Part model, mm, in its own coordinate system. Round coordinates to 2 decimals unless told otherwise and drop trailing zeros. Loops run counter-clockwise (first coordinate to the right, second up) from the corner with the lowest first, then second, coordinate; pieces in that order, holes last.
1) Probe line 1 (X direction, y = 1.2, z = 0); line 2 (Z direction, x = 2, y = 2.75); line 3 (X direction, y = 1.25, z = 5). List the from-to ranges inside material, lowest first.
2) Band-saw the part on C-C, the plane y = 2.5. State how many separate pieces and enclosed holes the cut face has, then the cut area to 3 significant figures.
3) Band-saw the part on A-A, the plane z = 0. Write the cut outline in (x, y).
4) Band-saw the part on D-D, the plane x = 30. Write the cut outline in (y, z).
5) Drop flat-ended pins along their axis: P1, Ø1, axis at y = 1, z = 8, coming from the -X side; P2, Ø0.9, axis at x = 87, y = 1.5, coming from the +Z side; P3, Ø0.9, axis at x = -1, y = 1, coming from the -Z side. Give the stop position or say it passes through.
6) Band-saw the part on B-B, the plane x = 0. Write the cut outline in (y, z), then the cut area to 3 significant figures.
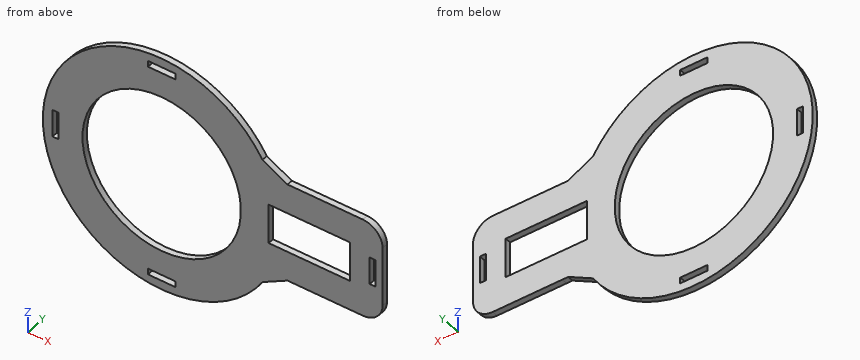
from build123d import *

# Parameters (mm, degrees)
EXTRUDE_1_DEPTH     = 3
SKETCH_3_W          = 13.8
SKETCH_3_H          = 3
SKETCH_3_W_2        = 3
SKETCH_3_H_2        = 13.8
CUT_EXTRUDE_1_DEPTH = 10
EXTRUDE_2_DEPTH     = 3
SKETCH_5_W          = 3
SKETCH_5_H          = 13.8
CUT_EXTRUDE_2_DEPTH = 20
SKETCH_6_W          = 41
SKETCH_6_H          = 20
CUT_EXTRUDE_3_DEPTH = 10
SKETCH_7_R          = 40
CUT_EXTRUDE_4_DEPTH = 3


with BuildPart() as part:
    # Эскиз2 → Бобышка-Вытянуть1 (new body)
    with BuildSketch(Plane(origin=(0, 0, 0), x_dir=(1, 0, 0), z_dir=(0, 1, 0))):
        with BuildLine():
            Line((50.901300831, -31.765666587), (63.52144012, -24.956238913))
            ThreePointArc((63.52144012, -24.956238913), (90, 0), (63.52144012, 24.956238913))
            Line((63.52144012, 24.956238913), (50.901300831, 31.765666587))
            ThreePointArc((50.901300831, 31.765666587), (-60, 0), (50.901300831, -31.765666587))
        make_face()
    extrude(amount=EXTRUDE_1_DEPTH)

    # Эскиз3 → Вырез-Вытянуть1 (cut)
    with BuildSketch(Plane(origin=(0, 3, 0), x_dir=(1, 0, 0), z_dir=(0, 1, 0))):
        with Locations((0, 53.956851754)):
            Rectangle(SKETCH_3_W, SKETCH_3_H)
        with Locations((0, -53.956851754)):
            Rectangle(SKETCH_3_W, SKETCH_3_H)
        with Locations((-53.60522772, 0)):
            Rectangle(SKETCH_3_W_2, SKETCH_3_H_2)
        with Locations((84.05982534, 0)):
            Rectangle(SKETCH_3_W_2, SKETCH_3_H_2)
    extrude(amount=-CUT_EXTRUDE_1_DEPTH, mode=Mode.SUBTRACT)

    # Эскиз4 → Бобышка-Вытянуть2 (add)
    with BuildSketch(Plane(origin=(0, 3, 0), x_dir=(1, 0, 0), z_dir=(0, 1, 0))):
        with BuildLine():
            Line((63.52144012, 24.956238913), (101.52144012, 24.956238913))
            ThreePointArc((101.52144012, 24.956238913), (108.592507932, 22.027306725), (111.52144012, 14.956238913))
            Line((111.52144012, 14.956238913), (111.52144012, -15))
            ThreePointArc((111.52144012, -15), (108.592507932, -22.071067812), (101.52144012, -25))
            Line((101.52144012, -25), (63.52144012, -25))
            Line((63.52144012, -25), (63.52144012, 24.956238913))
        make_face()
    extrude(amount=-EXTRUDE_2_DEPTH)

    # Эскиз5 → Вырез-Вытянуть2 (cut)
    with BuildSketch(Plane(origin=(0, 3, 0), x_dir=(1, 0, 0), z_dir=(0, 1, 0))):
        with Locations((106.52144012, -0.043761087)):
            Rectangle(SKETCH_5_W, SKETCH_5_H)
    extrude(amount=-CUT_EXTRUDE_2_DEPTH, mode=Mode.SUBTRACT)

    # Эскиз6 → Вырез-Вытянуть3 (cut)
    with BuildSketch(Plane(origin=(0, 3, 0), x_dir=(1, 0, 0), z_dir=(0, 1, 0))):
        with Locations((74.50144012, 0)):
            Rectangle(SKETCH_6_W, SKETCH_6_H)
    extrude(amount=-CUT_EXTRUDE_3_DEPTH, mode=Mode.SUBTRACT)

    # Эскиз7 → Вырез-Вытянуть4 (cut)
    with BuildSketch(Plane(origin=(0, 3, 0), x_dir=(1, 0, 0), z_dir=(0, 1, 0))):
        with Locations(Location((0, 0, 0), (0, 0, 270))):
            Circle(SKETCH_7_R)
    extrude(amount=-CUT_EXTRUDE_4_DEPTH, mode=Mode.SUBTRACT)


solid = part.part
Reported:
1. line 1: x = -60 to -55.11, -52.11 to -40, 40 to 54, 95 to 105.02, 108.02 to 111.52
1. line 2: z = -59.97 to -55.46, -52.46 to -39.95, 39.95 to 52.46, 55.46 to 59.97
1. line 3: x = -59.79 to -55.11, -52.11 to -39.69, 39.69 to 54, 95 to 105.02, 108.02 to 111.52
2. separate pieces: 1
2. enclosed holes: 6
2. area: 7,980 mm2
3. outline: (-60, 0) - (-55.11, 0) - (-55.11, 3) - (-60, 3) - close; (-52.11, 0) - (-40, 0) - (-40, 3) - (-52.11, 3) - close; (40, 0) - (54, 0) - (54, 3) - (40, 3) - close; (95, 0) - (105.02, 0) - (105.02, 3) - (95, 3) - close; (108.02, 0) - (111.52, 0) - (111.52, 3) - (108.02, 3) - close
4. outline: (0, -51.96) - (3, -51.96) - (3, -26.46) - (0, -26.46) - close; (0, 26.46) - (3, 26.46) - (3, 51.96) - (0, 51.96) - close
5. P1: stops at x = -59.53
5. P2: stops at z = 25
5. P3: stops at z = -60
6. outline: (0, -60) - (3, -60) - (3, -55.46) - (0, -55.46) - close; (0, -52.46) - (3, -52.46) - (3, -40) - (0, -40) - close; (0, 40) - (3, 40) - (3, 52.46) - (0, 52.46) - close; (0, 55.46) - (3, 55.46) - (3, 60) - (0, 60) - close
6. area: 102 mm2
